```python
from build123d import *

# Parameters (mm, degrees)
CYLINDER023_R     = 1
CYLINDER023_DEPTH = 9.5
SKETCH011_W       = 0.4
SKETCH011_H       = 0.4


with BuildPart() as part:
    # Cylinder023 → Cylinder023 (join)
    with BuildSketch(Plane.XY):
        Circle(CYLINDER023_R)
    extrude(amount=CYLINDER023_DEPTH)

    # Cone003 → Cone003 (revolve)
    with BuildSketch(Plane(origin=(0, 0, 9.3), x_dir=(1, 0, 0), z_dir=(0, -1, 0))):
        Polygon((0, 0), (1, 0), (1.75, 0.7), (0, 0.7), align=None)
    revolve(axis=Axis((0, 0, 9.3), (0, 0, 1)))

    # Sketch010 (on Face4 of Cone003) → SubtractiveLoft001 section 0
    with BuildSketch(Plane.XY.offset(10)):
        Polygon((-0.2, 0.2), (-0.2, 1.4), (0.2, 1.4), (0.2, 0.2), (1.4, 0.2), (1.4, -0.2), (0.2, -0.2), (0.2, -1.4), (-0.2, -1.4), (-0.2, -0.2), (-1.4, -0.2), (-1.4, 0.2), align=None)
    # Sketch011 (on Face4 of Cone003) → SubtractiveLoft001 section 1
    with BuildSketch(Plane.XY.offset(9)):
        Rectangle(SKETCH011_W, SKETCH011_H)
    loft(mode=Mode.SUBTRACT)


with BuildPart() as part_1:
    # Body011 placement: moved
    add(part.part.moved(Location((42.25, 30.5, -3.5))))


solid = part_1.part
```
CAD build for the part. Positions are in the model's coordinates, mm. A direction names the side the tool comes from. Round coordinates to 2 decimals unless told otherwise and drop trailing zeros. Write each loop counter-clockwise with the first axis right and the second up, starting at its lowest first coordinate (ties: lowest second). Pieces come first, ordered by that corner, then holes. Notation, with made-up numbers: (-35, 15.25) -> (-6, 15.25) arc R17 cw to (-6, 23.25) -> close; hole circle Ø3 at (10, -7). An arc over 180 degrees is marked (long way). Answer in a Markdown table with one row per item. Add a question column.
Item 1: Drill centre lines: line 1 (Z direction, x = 40.95, y = 31.05); line 2 (X direction, y = 31.2, z = -2.5); line 3 (Y direction, x = 41.45, z = 5.5). Where is each one in solid material? Low to high. Write a range as from..to.
Item 2: Drop a flat-ended pin along its axis: pin 1 Ø1.5 at (y, z) = (29.5, 3) entering from +X. Give the stop position or say it passes through.
Item 3: Saw through at A-A, the plane z = 2.25. Write the cut outline in (x, y).
Item 4: Which spindle directions (+Z, -Z, +X, -X, +Y, -Y) get a long thin tool onto all of the face, cutting with end or side? Do faces 1 (the face through (42.79, 31.34, 1.08)), 2 (the face through (42, 31, -3.5)). Say none if no direction does.
Findings below:
| question | item | result |
|---|---|---|
| 1 | line 1 | z = 6.18..6.5 |
| 1 | line 2 | x = 41.54..42.96 |
| 1 | line 3 | y = 29.9..31.1 |
| 2 | pin 1 | stops at x = 43.22 |
| 3 | outline | circle Ø2 at (42.25, 30.5) |
| 4 | face 1 | -Z |
| 4 | face 2 | -Z, +X, -X, +Y, -Y |
